Part model, mm, in its own coordinate system. Coordinates: 2 decimals unless noted, no trailing zeros. Order: outer loops, then holes, each group sorted by start corner. A loop starts at its lowest first (then second) coordinate and runs counter-clockwise, first axis right, second up.
```python
from build123d import *

# Parameters (mm, degrees)
SALIENTE_EXTRUIR1_DEPTH = 11
CROQUIS2_R              = 33
CROQUIS2_R_2            = 6.2
CORTAR_EXTRUIR1_DEPTH   = 10
SALIENTE_EXTRUIR2_DEPTH = 1
SALIENTE_EXTRUIR3_DEPTH = 10


with BuildPart() as part:
    # Croquis1 → Saliente-Extruir1 (new body)
    with BuildSketch(Plane.XY):
        with BuildLine():
            Line((-39.705480667, 55.513594064), (-58.980326234, 36.238748497))
            ThreePointArc((-58.980326234, 36.238748497), (-67.79562922, 41.581472229), (-77.806865921, 44.036956568))
            Line((-77.806865921, 44.036956568), (-77.806865921, 71.295704582))
            ThreePointArc((-77.806865921, 71.295704582), (-80.806865921, 85.669568124), (-83.806865921, 71.295704582))
            Line((-83.806865921, 71.295704582), (-83.806865921, 44.036956568))
            ThreePointArc((-83.806865921, 44.036956568), (-93.818102621, 41.581472229), (-102.633405607, 36.238748497))
            Line((-102.633405607, 36.238748497), (-121.908251174, 55.513594064))
            ThreePointArc((-121.908251174, 55.513594064), (-134.1934279, 63.556130104), (-126.150891861, 51.270953377))
            Line((-126.150891861, 51.270953377), (-106.876046294, 31.99610781))
            ThreePointArc((-106.876046294, 31.99610781), (-112.218770026, 23.180804824), (-114.674254364, 13.169568124))
            Line((-114.674254364, 13.169568124), (-141.933002378, 13.169568124))
            ThreePointArc((-141.933002378, 13.169568124), (-156.306865921, 10.169568124), (-141.933002378, 7.169568124))
            Line((-141.933002378, 7.169568124), (-114.674254364, 7.169568124))
            ThreePointArc((-114.674254364, 7.169568124), (-112.218770026, -2.841668576), (-106.876046294, -11.656971562))
            Line((-106.876046294, -11.656971562), (-126.150891861, -30.931817129))
            ThreePointArc((-126.150891861, -30.931817129), (-134.1934279, -43.216993856), (-121.908251174, -35.174457817))
            Line((-121.908251174, -35.174457817), (-102.633405607, -15.899612249))
            ThreePointArc((-102.633405607, -15.899612249), (-93.818102621, -21.242335981), (-83.806865921, -23.69782032))
            Line((-83.806865921, -23.69782032), (-83.806865921, -50.956568334))
            ThreePointArc((-83.806865921, -50.956568334), (-80.806865921, -65.330431876), (-77.806865921, -50.956568334))
            Line((-77.806865921, -50.956568334), (-77.806865921, -23.69782032))
            ThreePointArc((-77.806865921, -23.69782032), (-67.79562922, -21.242335981), (-58.980326234, -15.899612249))
            Line((-58.980326234, -15.899612249), (-39.705480667, -35.174457816))
            ThreePointArc((-39.705480667, -35.174457816), (-27.420303941, -43.216993856), (-35.46283998, -30.931817129))
            Line((-35.46283998, -30.931817129), (-54.737685547, -11.656971562))
            ThreePointArc((-54.737685547, -11.656971562), (-49.394961815, -2.841668576), (-46.939477477, 7.169568124))
            Line((-46.939477477, 7.169568124), (-19.680729463, 7.169568124))
            ThreePointArc((-19.680729463, 7.169568124), (-5.306865921, 10.169568124), (-19.680729463, 13.169568124))
            Line((-19.680729463, 13.169568124), (-46.939477477, 13.169568124))
            ThreePointArc((-46.939477477, 13.169568124), (-49.394961815, 23.180804824), (-54.737685547, 31.99610781))
            Line((-54.737685547, 31.99610781), (-35.46283998, 51.270953377))
            ThreePointArc((-35.46283998, 51.270953377), (-27.420303941, 63.556130104), (-39.705480667, 55.513594064))
        make_face()
    extrude(amount=SALIENTE_EXTRUIR1_DEPTH)

    # Croquis2 → Cortar-Extruir1 (cut)
    with BuildSketch(Plane.XY.offset(11)):
        with Locations((-80.806865921, 10.169568124)):
            Circle(CROQUIS2_R)
        with Locations((-128.890127041, 58.252829245)):
            Circle(CROQUIS2_R_2)
        with Locations((-80.806865921, 78.169568124)):
            Circle(CROQUIS2_R_2)
        with Locations((-32.7236048, 58.252829245)):
            Circle(CROQUIS2_R_2)
        with Locations((-12.806865921, 10.169568124)):
            Circle(CROQUIS2_R_2)
        with Locations((-32.7236048, -37.913692997)):
            Circle(CROQUIS2_R_2)
        with Locations((-80.806865921, -57.830431876)):
            Circle(CROQUIS2_R_2)
        with Locations((-128.890127041, -37.913692997)):
            Circle(CROQUIS2_R_2)
        with Locations((-148.806865921, 10.169568124)):
            Circle(CROQUIS2_R_2)
    extrude(amount=-CORTAR_EXTRUIR1_DEPTH, mode=Mode.SUBTRACT)

    # Croquis3 → Saliente-Extruir2 (add)
    with BuildSketch(Plane(origin=(0, 0, 0), x_dir=(-1, 0, 0), z_dir=(0, 0, -1))):
        with BuildLine():
            Line((114.674254364, 7.169568124), (141.933002378, 7.169568124))
            ThreePointArc((141.933002378, 7.169568124), (137.348025794, -13.250547128), (126.150891861, -30.931817129))
            Line((126.150891861, -30.931817129), (106.876046294, -11.656971562))
            ThreePointArc((106.876046294, -11.656971562), (112.218770026, -2.841668576), (114.674254364, 7.169568124))
        make_face()
        with BuildLine():
            Line((102.633405607, -15.899612249), (121.908251174, -35.174457816))
            ThreePointArc((121.908251174, -35.174457816), (104.226981172, -46.371591749), (83.806865921, -50.956568334))
            Line((83.806865921, -50.956568334), (83.806865921, -23.69782032))
            ThreePointArc((83.806865921, -23.69782032), (93.818102621, -21.242335981), (102.633405607, -15.899612249))
        make_face()
        with BuildLine():
            Line((77.806865921, -23.69782032), (77.806865921, -50.956568334))
            ThreePointArc((77.806865921, -50.956568334), (57.386750669, -46.371591749), (39.705480667, -35.174457816))
            Line((39.705480667, -35.174457816), (58.980326234, -15.899612249))
            ThreePointArc((58.980326234, -15.899612249), (67.79562922, -21.242335981), (77.806865921, -23.69782032))
        make_face()
        with BuildLine():
            Line((54.737685547, -11.656971562), (35.46283998, -30.931817129))
            ThreePointArc((35.46283998, -30.931817129), (24.265706047, -13.250547128), (19.680729463, 7.169568124))
            Line((19.680729463, 7.169568124), (46.939477477, 7.169568124))
            ThreePointArc((46.939477477, 7.169568124), (49.394961815, -2.841668576), (54.737685547, -11.656971562))
        make_face()
        with BuildLine():
            Line((46.939477477, 13.169568124), (19.680729463, 13.169568124))
            ThreePointArc((19.680729463, 13.169568124), (24.265706047, 33.589683376), (35.46283998, 51.270953377))
            Line((35.46283998, 51.270953377), (54.737685547, 31.99610781))
            ThreePointArc((54.737685547, 31.99610781), (49.394961815, 23.180804824), (46.939477477, 13.169568124))
        make_face()
        with BuildLine():
            Line((58.980326234, 36.238748497), (39.705480667, 55.513594064))
            ThreePointArc((39.705480667, 55.513594064), (57.386750669, 66.710727997), (77.806865921, 71.295704581))
            Line((77.806865921, 71.295704581), (77.806865921, 44.036956568))
            ThreePointArc((77.806865921, 44.036956568), (67.79562922, 41.581472229), (58.980326234, 36.238748497))
        make_face()
        with BuildLine():
            Line((83.806865921, 44.036956568), (83.806865921, 71.295704581))
            ThreePointArc((83.806865921, 71.295704581), (104.226981172, 66.710727997), (121.908251174, 55.513594064))
            Line((121.908251174, 55.513594064), (102.633405607, 36.238748497))
            ThreePointArc((102.633405607, 36.238748497), (93.818102621, 41.581472229), (83.806865921, 44.036956568))
        make_face()
        with BuildLine():
            Line((106.876046294, 31.99610781), (126.150891861, 51.270953377))
            ThreePointArc((126.150891861, 51.270953377), (137.348025794, 33.589683376), (141.933002378, 13.169568124))
            Line((141.933002378, 13.169568124), (114.674254364, 13.169568124))
            ThreePointArc((114.674254364, 13.169568124), (112.218770026, 23.180804824), (106.876046294, 31.99610781))
        make_face()
    extrude(amount=-SALIENTE_EXTRUIR2_DEPTH)

    # Croquis4 → Saliente-Extruir3 (add)
    with BuildSketch(Plane.XY.offset(1)):
        with BuildLine():
            Line((-126.150891861, -30.931817129), (-125.44378508, -30.224710348))
            ThreePointArc((-125.44378508, -30.224710348), (-136.425275383, -12.868331393), (-140.933002378, 7.169568124))
            Line((-140.933002378, 7.169568124), (-141.933002378, 7.169568124))
            ThreePointArc((-141.933002378, 7.169568124), (-137.348025794, -13.250547128), (-126.150891861, -30.931817129))
        make_face()
        with BuildLine():
            Line((-141.933002378, 13.169568124), (-140.933002378, 13.169568124))
            ThreePointArc((-140.933002378, 13.169568124), (-136.425275383, 33.207467641), (-125.44378508, 50.563846596))
            Line((-125.44378508, 50.563846596), (-126.150891861, 51.270953377))
            ThreePointArc((-126.150891861, 51.270953377), (-137.348025794, 33.589683376), (-141.933002378, 13.169568124))
        make_face()
        with BuildLine():
            Line((-121.908251174, 55.513594064), (-121.201144393, 54.806487283))
            ThreePointArc((-121.201144393, 54.806487283), (-103.844765438, 65.787977587), (-83.806865921, 70.295704581))
            Line((-83.806865921, 70.295704581), (-83.806865921, 71.295704581))
            ThreePointArc((-83.806865921, 71.295704581), (-104.226981172, 66.710727997), (-121.908251174, 55.513594064))
        make_face()
        with BuildLine():
            Line((-77.806865921, 71.295704581), (-77.806865921, 70.295704581))
            ThreePointArc((-77.806865921, 70.295704581), (-57.768966404, 65.787977587), (-40.412587448, 54.806487283))
            Line((-40.412587448, 54.806487283), (-39.705480667, 55.513594064))
            ThreePointArc((-39.705480667, 55.513594064), (-57.386750669, 66.710727997), (-77.806865921, 71.295704581))
        make_face()
        with BuildLine():
            Line((-35.46283998, 51.270953377), (-36.169946761, 50.563846596))
            ThreePointArc((-36.169946761, 50.563846596), (-25.188456458, 33.207467641), (-20.680729463, 13.169568124))
            Line((-20.680729463, 13.169568124), (-19.680729463, 13.169568124))
            ThreePointArc((-19.680729463, 13.169568124), (-24.265706047, 33.589683376), (-35.46283998, 51.270953377))
        make_face()
        with BuildLine():
            Line((-19.680729463, 7.169568124), (-20.680729463, 7.169568124))
            ThreePointArc((-20.680729463, 7.169568124), (-25.188456458, -12.868331393), (-36.169946761, -30.224710348))
            Line((-36.169946761, -30.224710348), (-35.46283998, -30.931817129))
            ThreePointArc((-35.46283998, -30.931817129), (-24.265706047, -13.250547128), (-19.680729463, 7.169568124))
        make_face()
        with BuildLine():
            Line((-39.705480667, -35.174457816), (-40.412587448, -34.467351035))
            ThreePointArc((-40.412587448, -34.467351035), (-57.768966404, -45.448841339), (-77.806865921, -49.956568334))
            Line((-77.806865921, -49.956568334), (-77.806865921, -50.956568334))
            ThreePointArc((-77.806865921, -50.956568334), (-57.386750669, -46.371591749), (-39.705480667, -35.174457816))
        make_face()
        with BuildLine():
            Line((-83.806865921, -50.956568334), (-83.806865921, -49.956568334))
            ThreePointArc((-83.806865921, -49.956568334), (-103.844765438, -45.448841339), (-121.201144393, -34.467351035))
            Line((-121.201144393, -34.467351035), (-121.908251174, -35.174457816))
            ThreePointArc((-121.908251174, -35.174457816), (-104.226981172, -46.371591749), (-83.806865921, -50.956568334))
        make_face()
    extrude(amount=SALIENTE_EXTRUIR3_DEPTH)


solid = part.part
```
(1) Drop flat-ended pins along their axis: pin 1 (5 mm diameter, centred on x = -39.5, z = 8.5, fed in from +Y); pin 2 (10 mm diameter, centred on x = -128.89, y = 58.25, fed in from +Z); pin 3 (6 mm diameter, centred on x = -116, z = 9, fed in from -Y). Give the stop position or say it passes through.
(2) Slice it at C-C, the plane z = 4.25. State how many separate pieces and enclosed holes the cut face has, then the cut area to 3 significant figures.
(3) Slice it at B-B, the plane y = 48. Give the cut face in (x, z), then the cut area to 3 significant figures.
(4) Slice it at D-D, the plane y = -28. Give the cut face in (x, z).
(5) Probe line 1 (X direction, y = -31, z = 1.75); line 2 (Y direction, x = -72.5, z = 1.75); line 3 (Y direction, x = -36.5, z = 2). List the from-to ranges inside material, lowest first.
(6) Slice it at A-A, the plane x = -146. Give the cut face in (y, z).
Here are the results:
1. pin 1: stops at y = 64.41
1. pin 2: stops at z = 1
1. pin 3: stops at y = -41.88
2. separate pieces: 1
2. enclosed holes: 17
2. area: 2,280 mm2
3. outline: (-128.91, 0) - (-32.7, 0) - (-32.7, 11) - (-33.98, 11) - (-33.98, 1) - (-38.73, 1) - (-38.73, 11) - (-47.22, 11) - (-47.22, 1) - (-77.81, 1) - (-77.81, 11) - (-83.81, 11) - (-83.81, 1) - (-114.39, 1) - (-114.39, 11) - (-122.88, 11) - (-122.88, 1) - (-127.64, 1) - (-127.64, 11) - (-128.91, 11) - close
3. area: 351 mm2
4. outline: (-128.65, 0) - (-32.97, 0) - (-32.97, 11) - (-34.25, 11) - (-34.25, 1) - (-38.39, 1) - (-38.39, 11) - (-46.88, 11) - (-46.88, 1) - (-77.81, 1) - (-77.81, 11) - (-83.81, 11) - (-83.81, 1) - (-114.73, 1) - (-114.73, 11) - (-123.22, 11) - (-123.22, 1) - (-127.36, 1) - (-127.36, 11) - (-128.65, 11) - close
5. line 1: x = -131.8 to -117.73, -83.81 to -77.81, -43.88 to -29.82
5. line 2: y = -50.46 to -49.46, -22.8 to -21.77, 42.11 to 43.14, 69.79 to 70.8
5. line 3: y = -44.39 to -42.83, -33 to -29.89, 7.17 to 13.17, 50.23 to 53.34, 63.17 to 64.73
6. outline: (3.21, 0) - (17.12, 0) - (17.12, 11) - (15.7, 11) - (15.7, 1) - (4.64, 1) - (4.64, 11) - (3.21, 11) - close
